Source: CAD feature listing. Evaluate the final solid. Frame: model axes, mm. A direction names the side the tool comes from. Give positions to 0.01 mm unless a question says otherwise; leave off trailing zeros. Order: outer loops, then holes, each group sorted by start corner. A loop starts at its lowest first (then second) coordinate and runs counter-clockwise, first axis right, second up. Notation, with made-up numbers: (57.5, -15) -> (106.5, -15) arc R12 ccw to (106.5, 3) -> close; hole circle Ø8 at (75.25, 5). An arc over 180 degrees is marked (long way). Answer in a Markdown table with one row per item.
```python
from build123d import *

# Parameters (mm, degrees)
F1_ANGLE_BACK = 45
F1_ANGLE      = 90


# Not quite as in the source:
# - a feature of the source that left no trace in its solid (it failed there, or was rolled back) is left out


with BuildPart() as f1:
    # F0 (on Front) → F1 (revolve)
    with BuildSketch(Plane.XZ, mode=Mode.PRIVATE) as f1_sk:
        Polygon((0, 40), (-25, 40), (-25, 30), (-35, 30), (-35, 10), (-18, 10), (-18, -5.7214838854), (-35, -30), (0, -30), align=None)
    revolve(f1_sk.sketch.rotate(Axis((0, 0, 5), (0, 0, 1)), -F1_ANGLE_BACK), axis=Axis((0, 0, 5), (0, 0, 1)), revolution_arc=F1_ANGLE)


solid = f1.part
```
(1) Section query C-C (x = -7.5). Return the cut outline in (y, z), plus the area to 3 significant figures.
A:
| item | result |
|---|---|
| outline | (-7.5, -30) -> (7.5, -30) -> (7.5, 40) -> (-7.5, 40) -> close |
| area | 1,050 mm^2 |
(2) First-contact query: pin 1 Ø8 at (y, z) = (-10.5, -9.5) entering from -X; pin 2 Ø10 at (y, z) = (12.5, 13) entering from +X; pin 3 Ø5 at (x, z) = (-15, -6) entering from -Y. Flat tips, straight axial feed; report the tip coordinate or a pass-through.
A:
| item | result |
|---|---|
| pin 1 | stops at x = -21.45 |
| pin 2 | stops at x = -7.5 |
| pin 3 | stops at y = -14 |
(3) Section query A-A (x = -3.5). Return the cut outline in (y, z).
A:
| item | result |
|---|---|
| outline | (-3.5, -30) -> (3.5, -30) -> (3.5, 40) -> (-3.5, 40) -> close |
(4) Pull-direction query (Z, two-part tool) for faces 1 (the flat face through (-14, 0, 40)), 2 (the flat face through (-25, 0, 10)), 3 (the flat face through (-19, 0, -30)), 4 (the conical face through (-26.617, 0.293, -18.031)); classes: +Z half, -Z half, draft (parallel to the pull), parting line (faces both ways), or undercut.
A:
| item | result |
|---|---|
| face 1 | +Z half |
| face 2 | undercut |
| face 3 | -Z half |
| face 4 | undercut |
(5) Section query B-B (z = 26). Return the cut outline in (x, y).
A:
| item | result |
|---|---|
| outline | (-24.75, -24.75) -> (0, 0) -> (-24.75, 24.75) arc R35 ccw to start |
(6) Access query for faces 5 (the cylindrical face through (-35, 0, 20)), 6 (the cylindrical face through (-18, 0, 2)), 7 (the cylindrical face through (-25, 0, 35)). Directions: +Z, -Z, +X, -X, +Y, -Y. A direction counts if a zero-diameter tool reaches every point of the face in a straight line with its end or side. Return the directions, or none.
A:
| item | result |
|---|---|
| face 5 | +Z, -Z, -X |
| face 6 | -X |
| face 7 | +Z, -X |
(7) Section query D-D (z = -18). Return the cut outline in (x, y), plus the area to 3 significant figures.
A:
| item | result |
|---|---|
| outline | (-18.81, -18.81) -> (0, 0) -> (-18.81, 18.81) arc R26.6 ccw to start |
| area | 556 mm^2 |
(8) Ray query, probe 1 along Z at (x, y) = (-18, 14.5); probe 2 along Z at (x, y) = (-26, 7); probe 3 along Y at (x, z) = (-23.5, -17). Return the intervals inside material, ascending.
A:
| item | result |
|---|---|
| probe 1 | z = -30 to -13.02, 10 to 40 |
| probe 2 | z = -30 to -18.47, 10 to 30 |
| probe 3 | y = -10.88 to 10.88 |
